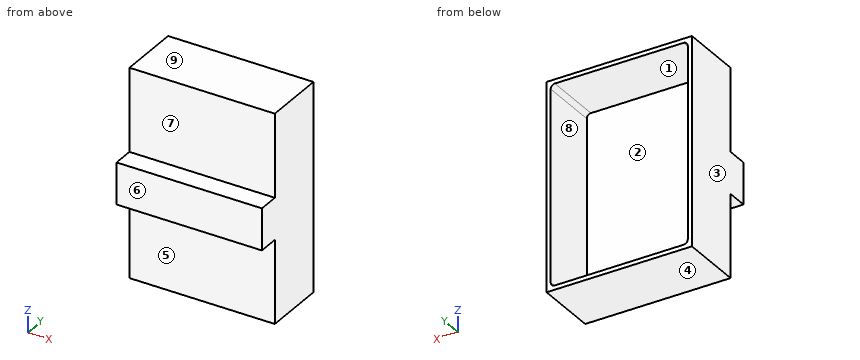
from build123d import *

# Parameters (mm, degrees)
BOSS_EXTRUDE1_DEPTH        = 70
SHELL16_T                  = -2
SHELL16_THICKNESS_2_FACE_W = 16
SHELL16_THICKNESS_2_FACE_H = 66
SHELL16_THICKNESS_2_DEPTH  = 10
FILLET1_R                  = 2


with BuildPart() as part:
    # Sketch1 → Boss-Extrude1 (new body)
    with BuildSketch(Plane(origin=(0, 0, 0), x_dir=(0, 0, -1), z_dir=(1, 0, 0))):
        Polygon((40, 0), (60, 0), (60, 10), (100, 10), (100, 40), (0, 40), (0, 10), (40, 10), align=None)
    extrude(amount=BOSS_EXTRUDE1_DEPTH)

    # Shell16
    shell16_openings = [part.faces().sort_by_distance(p)[0] for p in [
        (35, 40, -50),
    ]]
    offset(amount=SHELL16_T, openings=shell16_openings, kind=Kind.INTERSECTION)

    # Shell16 thickness 2 face (on inner face of the shell) → Shell16 thickness 2 (add)
    with BuildSketch(Plane(origin=(35, 2, -50), x_dir=(0, 0, -1), z_dir=(0, -1, 0))):
        Rectangle(SHELL16_THICKNESS_2_FACE_W, SHELL16_THICKNESS_2_FACE_H)
    extrude(amount=-SHELL16_THICKNESS_2_DEPTH)

    # Fillet1
    fillet1_edges = [part.edges().sort_by_distance(p)[0] for p in [
        (2, 26, -98),
        (2, 26, -2),
        (68, 26, -98),
        (68, 26, -2),
    ]]
    fillet(fillet1_edges, radius=FILLET1_R)


solid = part.part
Model file for the job. Use its own axes, mm. Face numbers are marked on the shaded views. A direction names the side the tool comes from. Round coordinates to 2 decimals unless told otherwise and drop trailing zeros. Order: outer loops, then holes, each group sorted by start corner. A loop starts at its lowest first (then second) coordinate and runs counter-clockwise, first axis right, second up. Notation, with made-up numbers: M -33.75,76 L -12.75,76 A6 cw -12.75,85 Z; hole C 50.25,-35 d8. An arc over 180 degrees is marked long. Write each question's results on one line, items separated by ' | '. Start each with the question number.
(1) Probe probe 1 along X at (y, z) = (21, -29); probe 2 along Z at (x, y) = (59, 22.5); probe 3 along Z at (x, y) = (28, 7). List the from-to ranges inside material, lowest first. Write a range as from..to.
(2) Saw through at A-A, the plane y = 15. Give the cut face in (x, z), then the cut area to 3 significant figures.
(3) Two-plate mould, pull along Z, no slides. Class the marked faces 1, 2, 3 and 4: pulls with the +Z half, pulls with the -Z half, needs draft (parallel to the pull), parting line crosses it, or undercut.
(4) Saw through at B-B, the plane x = 32. Give the cut face in (y, z), then the cut area to 3 significant figures.
(5) Drop flat-ended pins along their axis: pin 1 (20 mm diameter, centred on x = 27.5, z = -81.5, fed in from -Y); pin 2 (10 mm diameter, centred on y = 4, z = -26.5, fed in from +X); pin 3 (3 mm diameter, centred on x = 42, z = -90, fed in from +Y); pin 4 (5 mm diameter, centred on x = 40.5, y = 7, fed in from +Z). Give the stop position or say it passes through.
(6) Saw through at C-C, the plane z = -74.5. Give the cut face in (x, y).
(7) Which spindle directions (+Z, -Z, +X, -X, +Y, -Y) get a long thin tool onto all of the face, cutting with end or side? Do the marked faces 5, 6, 7, 8 and 9. Say none if no direction does.
Established:
1) probe 1: x = 0..2, 68..70 | probe 2: z = -100..-98, -2..0 | probe 3: z = -60..-40
2) outline: M 0,-100 L 70,-100 L 70,0 L 0,0 Z; hole M 2,-96 A2 ccw 4,-98 L 66,-98 A2 ccw 68,-96 L 68,-4 A2 ccw 66,-2 L 4,-2 A2 ccw 2,-4 Z | area: 667 mm^2
3) face 1: undercut | face 2: undercut | face 3: needs draft | face 4: pulls with the -Z half
4) outline: M 0,-60 L 10,-60 L 10,-100 L 40,-100 L 40,-98 L 12,-98 L 12,-2 L 40,-2 L 40,0 L 10,0 L 10,-40 L 0,-40 Z | area: 512 mm^2
5) pin 1: stops at y = 10 | pin 2: passes through | pin 3: stops at y = 12 | pin 4: stops at z = -40
6) outline: M 0,10 L 70,10 L 70,40 L 68,40 L 68,12 L 2,12 L 2,40 L 0,40 Z
7) face 5: -Z, +X, -X, -Y | face 6: +Z, -Z, +X, -X, -Y | face 7: +Z, +X, -X, -Y | face 8: +Y | face 9: +Z, +X, -X, +Y, -Y
